Part print with two shaded views. Sizes in mm from the minimum x, y, z corner. Give positions to 0.01 mm unless a question says otherwise; leave off trailing zeros. Order: outer loops, then holes, each group sorted by start corner. A loop starts at its lowest first (then second) coordinate and runs counter-clockwise, first axis right, second up. Notation, with made-up numbers: (4.25, 18.25) -> (30.25, 18.25) arc R24 cw to (30.25, 44.25) -> close; hole circle Ø7 at (19.25, 24). An arc over 180 degrees is marked (long way). Write item = value, one per line. Start each with the question number.
Item 1: Flat gauge pin, fed straight in: P1, Ø4.5, axis at x = 109.474, y = 9.525, coming from the +Z side. Where does the tip first touch, or does it go through?
Item 2: Band-saw the part on B-B on z = 7. Write the cut outline in (x, y) (3 decimals).
Item 3: Drill centre lines: line 1 along X through (y, z) = (9, 3); line 2 along X through (y, z) = (1, 5.5); line 3 along X through (y, z) = (7, 12). Where is each one in solid material? Low to high.
Item 4: Band-saw the part on A-A on x = 25.4. Write the cut outline in (y, z), plus the area to 4 significant figures.
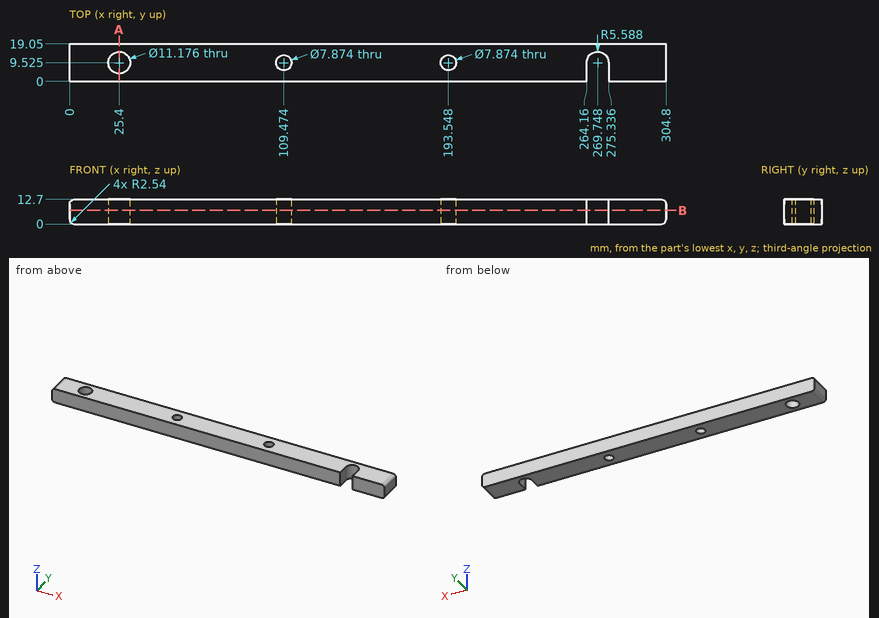
Values found:
q1.P1 = through
q2.outline = (0, 0) -> (264.16, 0) -> (264.16, 9.525) arc R5.588 cw to (275.336, 9.525) -> (275.336, 0) -> (304.8, 0) -> (304.8, 19.05) -> (0, 19.05) -> close; hole circle Ø11.176 at (25.4, 9.525); hole circle Ø7.874 at (109.474, 9.525); hole circle Ø7.874 at (193.548, 9.525)
q3.line_1 = 0 to 19.84, 30.96 to 105.57, 113.38 to 189.65, 197.45 to 264.16, 275.34 to 304.8
q3.line_2 = 0 to 264.16, 275.34 to 304.8
q3.line_3 = 0.79 to 20.42, 30.38 to 106.45, 112.49 to 190.53, 196.57 to 264.16, 275.34 to 304.01
q4.outline = (0, 0) -> (3.94, 0) -> (3.94, 12.7) -> (0, 12.7) -> close; (15.11, 0) -> (19.05, 0) -> (19.05, 12.7) -> (15.11, 12.7) -> close
q4.area = 100.0 mm^2
